Autodesk Inventor part; units mm, degrees
ref_plane "YZ Plane" through (0, 0, 0) normal (1, 0, 0) x (0, 1, 0)
ref_plane "XZ Plane" through (0, 0, 0) normal (0, 1, 0) x (-1, 0, 0)
ref_plane "XY Plane" through (0, 0, 0) normal (0, 0, 1) x (1, 0, 0)
sketch "Sketch1" plane through (0, 0, 0) normal (0, 0, 1) x (1, 0, 0)
  line L0 (0, 0) -> (25.4, 0)
  line L1 (25.4, 0) -> (25.4, 50.8)
  line L2 (25.4, 50.8) -> (0, 50.8)
  line L3 (0, 50.8) -> (0, 0)
  line L4 (22.225, 3.175) -> (3.175, 3.175)
  line L5 (3.175, 3.175) -> (3.175, 47.625)
  line L6 (3.175, 47.625) -> (22.225, 47.625)
  line L7 (22.225, 47.625) -> (22.225, 3.175)
  dimension "d0" = 25.4
  dimension "d1" = 50.8
  dimension "d2" = 3.175
  dimension "d3" = 3.175
  dimension "d4" = 3.175
  dimension "d5" = 3.175
extrude "Extrusion1" add sketch "Sketch1" along normal blind 228.6
sketch "Sketch2" plane through (0, 0, 0) normal (-1, 0, 0) x (0, 0, 1)
  circle A0 centre (215.9, 38.1) radius 3.3734
  circle A1 centre (190.5, 38.1) radius 3.3734
  line L0 (0, 50.8) -> (228.6, 50.8)
  line L1 (228.6, 50.8) -> (228.6, 0)
  point P0 (0, 0)
  dimension "d8" = 6.7469
  dimension "d9" = 6.7469
  dimension "d10" = 12.7
  dimension "d11" = 12.7
  dimension "d12" = 12.7
  dimension "d13" = 38.1
extrude "Extrusion2" cut sketch "Sketch2" against normal blind 25.4
properties part number "superstructure" material "Aluminum 6061"
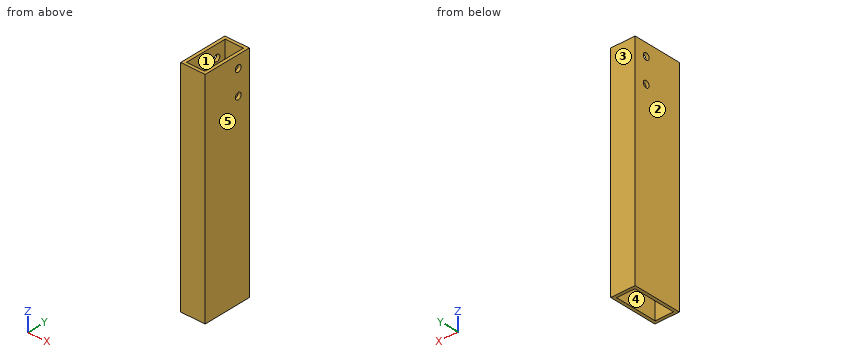
The listing builds one solid part. Answer for the finished solid, in the listing's coordinates (mm). Face numbers are marked on the shaded views. A direction names the side the tool comes from. Coordinates: 2 decimals unless noted, no trailing zeros. Loops run counter-clockwise (first coordinate to the right, second up) from the corner with the lowest first, then second, coordinate; pieces in that order, holes last. Notation, with made-up numbers: M -20.75,-9 L 11.25,-9 A34 ccw 11.25,23 Z; hole C 64,1 d3. An arc over 180 degrees is marked long. Answer in a Markdown table with one row per item.
1) Find section A-A (y = 26). Determine the outline of the cut face in (x, z) (3 decimals).
Answers below:
| item | result |
|---|---|
| outline | M 0,0 L 3.175,0 L 3.175,228.6 L 0,228.6 Z; M 22.225,0 L 25.4,0 L 25.4,228.6 L 22.225,228.6 Z |
2) Find the intervals of material crossed by probe 1 along X at (y, z) = (41, 142.5) (3 decimals); probe 2 along Y at (x, z) = (24.25, 190.5); probe 3 along Y at (x, z) = (19, 29.5) (3 decimals), in increasing order.
Answers below:
| item | result |
|---|---|
| probe 1 | 0 to 3.175, 22.225 to 25.4 |
| probe 2 | 0 to 34.73, 41.47 to 50.8 |
| probe 3 | 0 to 3.175, 47.625 to 50.8 |
3) Find section D-D (y = 38.1). Determine the outline of the cut face in (x, z) (3 decimals), then the cut area to 3 significant figures.
Answers below:
| item | result |
|---|---|
| outline | M 0,0 L 3.175,0 L 3.175,187.127 L 0,187.127 Z; M 0,193.873 L 3.175,193.873 L 3.175,212.527 L 0,212.527 Z; M 0,219.273 L 3.175,219.273 L 3.175,228.6 L 0,228.6 Z; M 22.225,0 L 25.4,0 L 25.4,187.127 L 22.225,187.127 Z; M 22.225,193.873 L 25.4,193.873 L 25.4,212.527 L 22.225,212.527 Z; M 22.225,219.273 L 25.4,219.273 L 25.4,228.6 L 22.225,228.6 Z |
| area | 1,370 mm^2 |
4) Given pin 1 (5.5 mm diameter, centred on y = 38.1, z = 190.5, fed in from +X), flat-ended and moving along its own axis, determine where the tip first touches the part or whether it passes through.
Answers below:
| item | result |
|---|---|
| pin 1 | through |
5) Find section C-C (x = 6.5). Determine the outline of the cut face in (y, z) (3 decimals), then the cut area to 3 significant figures.
Answers below:
| item | result |
|---|---|
| outline | M 0,0 L 3.175,0 L 3.175,228.6 L 0,228.6 Z; M 47.625,0 L 50.8,0 L 50.8,228.6 L 47.625,228.6 Z |
| area | 1,450 mm^2 |
6) Find section B-B (z = 190.5). Determine the outline of the cut face in (x, y) (3 decimals), then the cut area to 3 significant figures.
Answers below:
| item | result |
|---|---|
| outline | M 0,0 L 25.4,0 L 25.4,34.727 L 22.225,34.727 L 22.225,3.175 L 3.175,3.175 L 3.175,34.727 L 0,34.727 Z; M 0,41.473 L 3.175,41.473 L 3.175,47.625 L 22.225,47.625 L 22.225,41.473 L 25.4,41.473 L 25.4,50.8 L 0,50.8 Z |
| area | 401 mm^2 |
7) Determine the mould class of the marked faces 3, 4 and 5 for opening direction X: released by +X, released by -X, zero draft, split by the parting line, or undercut.
Answers below:
| item | result |
|---|---|
| face 3 | zero draft |
| face 4 | undercut |
| face 5 | released by +X |
8) Which of the six approach directions +Z, -Z, +X, -X, +Y, -Y give full straight-line access (tool end or side, diameter ignored) to the marked faces 1 and 2?
Answers below:
| item | result |
|---|---|
| face 1 | +Z, -Z |
| face 2 | +Z, -Z, -X, +Y, -Y |
